Answer from the drawing. Dimensions are ordinates in mm from the lowest x, y and z of the part. A direction names the side the tool comes from. Coordinates: 2 decimals unless noted, no trailing zeros. Write each loop counter-clockwise with the first axis right and the second up, starting at its lowest first coordinate (ties: lowest second). Pieces come first, ordered by that corner, then holes. Notation, with made-up numbers: M 33,-3.5 L 66,-3.5 A19 cw 66,0.5 Z; hole C -7.5,16.5 d9. An arc over 180 degrees is marked long. Put each result on its own line as item: value. Start each with the question number.
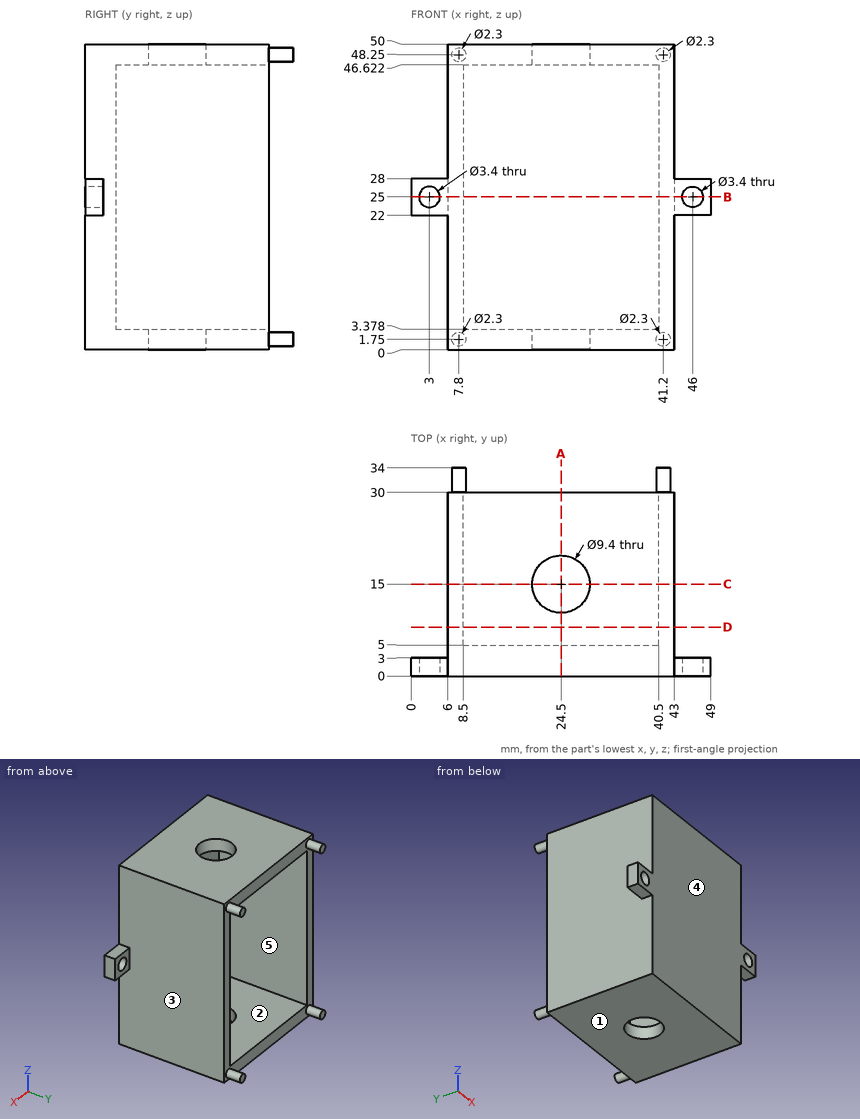
1) A cutting plane is placed at C-C on y = 15. Write down the section's boundary in (x, z).
2) Given pin 1 Ø3.5 at (x, y) = (3.5, 1) entering from +Z; pin 2 Ø20 at (x, y) = (26, 12.5) entering from +Z; pin 3 Ø8 at (x, z) = (21, 30.5) entering from +Y; pin 4 Ø7.5 at (y, z) = (20.5, 31) entering from -X, each flat-ended and moving along its own axis, determine where each tip first touches the part or whether it passes through.
3) Straight lines are drawn through the part: probe 1 along X at (y, z) = (1.4, 25); probe 2 along Z at (x, y) = (46, 1); probe 3 along Z at (x, y) = (13, 12). For each, find the intervals that lie inside material, in ascending order.
4) For the marked faces 4 and 5, determine the directions among +Z, -Z, +X, -X, +Y, -Y from which every point of the face is accessible in a straight line to the end or side of a thin tool.
5) A cutting plane is placed at D-D on y = 8. Write down the section's boundary in (x, z).
6) Determine the mould class of the marked faces 1, 2 and 3 for opening direction Z: +Z half, -Z half, draft (parallel to the pull), parting line (faces both ways), or undercut.
7) A cutting plane is placed at A-A on x = 24.5. Write down the section's boundary in (y, z).
8) A cutting plane is placed at B-B on z = 25. Write down the section's boundary in (x, y).
Answers follow:
1. outline: M 6,0 L 19.8,0 L 19.8,3.38 L 8.5,3.38 L 8.5,46.62 L 19.8,46.62 L 19.8,50 L 6,50 Z; M 29.2,0 L 43,0 L 43,50 L 29.2,50 L 29.2,46.62 L 40.5,46.62 L 40.5,3.38 L 29.2,3.38 Z
2. pin 1: stops at z = 28
2. pin 2: stops at z = 50
2. pin 3: stops at y = 5
2. pin 4: stops at x = 6
3. probe 1: x = 0 to 1.3, 4.7 to 44.3, 47.7 to 49
3. probe 2: z = 22 to 23.3, 26.7 to 28
3. probe 3: z = 0 to 3.38, 46.62 to 50
4. face 4: +Z, -Z, +X, -X, -Y
4. face 5: +Y
5. outline: M 6,0 L 43,0 L 43,50 L 6,50 Z; hole M 8.5,3.38 L 40.5,3.38 L 40.5,46.62 L 8.5,46.62 Z
6. face 1: -Z half
6. face 2: undercut
6. face 3: draft
7. outline: M 0,0 L 10.3,0 L 10.3,3.38 L 5,3.38 L 5,46.62 L 10.3,46.62 L 10.3,50 L 0,50 Z; M 19.7,0 L 30,0 L 30,3.38 L 19.7,3.38 Z; M 19.7,46.62 L 30,46.62 L 30,50 L 19.7,50 Z
8. outline: M 0,0 L 1.3,0 L 1.3,3 L 0,3 Z; M 4.7,0 L 44.3,0 L 44.3,3 L 43,3 L 43,30 L 40.5,30 L 40.5,5 L 8.5,5 L 8.5,30 L 6,30 L 6,3 L 4.7,3 Z; M 47.7,0 L 49,0 L 49,3 L 47.7,3 Z
